Geometry check sheet. Reference: drawing and pictorial views, mm from the part's lowest x, y, z. A direction names the side the tool comes from. Round coordinates to 2 decimals unless told otherwise and drop trailing zeros. Order: outer loops, then holes, each group sorted by start corner. A loop starts at its lowest first (then second) coordinate and runs counter-clockwise, first axis right, second up. Notation, with made-up numbers: (1, 33) -> (23, 33) arc R22 cw to (23, 65) -> close; hole circle Ø4 at (37, 60). An arc over 180 degrees is marked (long way). Put each result on its own line as item: value.
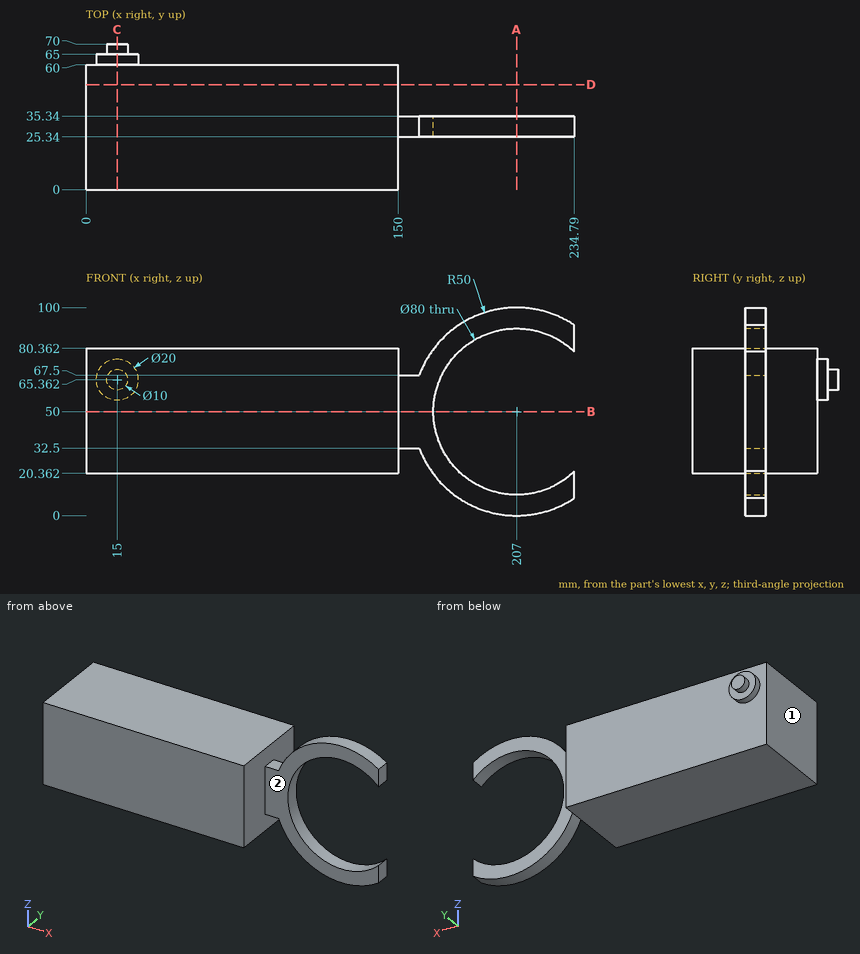
Item 1: Material ranges on line 1 along Z through (x, y) = (207, 31); line 2 along Z through (x, y) = (82.5, 25); line 3 along X through (y, z) = (11.5, 48.5), recorded low to high.
Geometry check:
line 1: 0 to 10, 90 to 100
line 2: 20.36 to 80.36
line 3: 0 to 150
Item 2: Tool access check on the marked faces 1 and 2. Record the directions out of +Z, -Z, +X, -X, +Y, -Y that give a thin tool (end or side, any length) a straight path to the whole face; none if there is none.
Geometry check:
face 1: +Z, -Z, -X, +Y, -Y
face 2: +Z, -Z, +X, -Y
Item 3: Depth check by flat-ended pin: pin 1 Ø2 at (y, z) = (41.5, 82) entering from +X; pin 2 Ø6 at (x, y) = (139, 17) entering from +Z; pin 3 Ø11 at (x, y) = (156, 32.5) entering from +Z; pin 4 Ø1.5 at (y, z) = (22.5, 69.5) entering from +X. Enter the tip coordinate at first touch or a pass-through.
Geometry check:
pin 1: through
pin 2: z = 80.36
pin 3: z = 70.73
pin 4: x = 150
Item 4: Sectioned sample at C-C, the plane x = 15. Record the boundary of the cut face in (y, z), then the cut area to 3 significant figures.
Geometry check:
outline: (0, 20.36) -> (60, 20.36) -> (60, 55.36) -> (65, 55.36) -> (65, 60.36) -> (70, 60.36) -> (70, 70.36) -> (65, 70.36) -> (65, 75.36) -> (60, 75.36) -> (60, 80.36) -> (0, 80.36) -> close
area: 3,750 mm2
Item 5: Sectioned sample at D-D, the plane y = 50.5. Record the boundary of the cut face in (x, z), then the cut area to 3 significant figures.
Geometry check:
outline: (0, 20.36) -> (150, 20.36) -> (150, 80.36) -> (0, 80.36) -> close
area: 9,000 mm2
Item 6: Sectioned sample at B-B, the plane z = 50. Record the boundary of the cut face in (x, y), then the cut area to 3 significant figures.
Geometry check:
outline: (0, 0) -> (150, 0) -> (150, 25.34) -> (167, 25.34) -> (167, 35.34) -> (150, 35.34) -> (150, 60) -> (0, 60) -> close
area: 9,170 mm2
Item 7: Sectioned sample at A-A, the plane x = 207. Record the boundary of the cut face in (y, z).
Geometry check:
outline: (25.34, 0) -> (35.34, 0) -> (35.34, 10) -> (25.34, 10) -> close; (25.34, 90) -> (35.34, 90) -> (35.34, 100) -> (25.34, 100) -> close
